Read the model definition and answer for the solid it produces. Units are mm, in the model's axes. A direction names the side the tool comes from. Coordinates: 2 decimals unless noted, no trailing zeros. Loops run counter-clockwise (first coordinate to the right, second up) from the corner with the lowest first, then second, coordinate; pieces in that order, holes last. Notation, with made-up numbers: (55, 74.25) -> (99, 74.25) arc R21 ccw to (99, 105.25) -> close; hole circle Ø4 at (2, 87). An arc over 180 degrees is marked (long way). Answer as a JSON object with one key per item and string values. Group by question number.
1) Section D-D, the plane x = 0 is taken. Give the vertices of the cut face in (y, z) (3 decimals).
2) Section C-C, the plane x = 30 is taken. Give the vertices of the cut face in (y, z).
3) Consider probe 1 along X at (y, z) = (27, 2.5); probe 2 along X at (y, z) = (0.5, 4); probe 3 along Y at (x, z) = (33.5, 5.25). Determine where each line is inside the solid, lowest interval first. Write a range as [from, to].
4) Which of the six approach directions +Z, -Z, +X, -X, +Y, -Y give full straight-line access (tool end or side, diameter ignored) to faces 4 (the face through (-3, -43, 0)), 5 (the face through (34.29, 39, 3)), 6 (the face through (-31, -38.1, 3)), 7 (the face through (31.75, 39, 3)), 8 (the face through (33, 43, 3.94))?
5) Section B-B, the plane z = 2 is taken. Count the separate pieces of the cut face and the enclosed holes in it, plus the area to 3 significant figures.
6) Determine the mould class of faces 1 (the face through (31, -38.1, 3)), 2 (the face through (38.1, -41, 3)), 3 (the face through (-1, -44.45, 3)) for opening direction Y: released by +Y, released by -Y, zero draft, split by the parting line, or undercut.
7) Flat-ended cylindrical pins translate along their axes: P1, Ø2, axis at y = -7.5, z = 2, coming from the +X side; P2, Ø3, axis at y = 45, z = 2.5, coming from the +X side; P3, Ø2, axis at y = 4, z = 4, coming from the -X side; P4, Ø1, axis at x = -2, z = 4.5, coming from the +Y side. Find the tip coordinate at first contact, or state that the pin passes through.
from build123d import *

# Parameters (mm, degrees)
SKETCH1_R            = 41.275
BOSS_EXTRUDE1_DEPTH  = 6.35
FILLET1_R            = 1.27
SKETCH2_W            = 63.5
SKETCH2_H            = 38.1
CUT_EXTRUDE1_DEPTH   = 6.35
SKETCH3_W            = 6.35
SKETCH3_H            = 25.4
BOSS_EXTRUDE2_DEPTH  = 2.54
FILLET2_R            = 1.27
FILLET2_OF_MIRROR1_R = 1.27
SKETCH6_R            = 2.54
CUT_EXTRUDE2_DEPTH   = 93.605338907


with BuildPart() as part:
    # Sketch1 → Boss-Extrude1 (new body)
    with BuildSketch(Plane.XY):
        with BuildLine():
            Line((-18.208562718, -38.1), (-38.1, -38.1))
            Line((-38.1, -38.1), (-38.1, -44.45))
            Line((-38.1, -44.45), (38.1, -44.45))
            Line((38.1, -44.45), (38.1, -38.1))
            Line((38.1, -38.1), (18.208562718, -38.1))
            ThreePointArc((18.208562718, -38.1), (0, 42.2275), (-18.208562718, -38.1))
        make_face()
        Circle(SKETCH1_R, mode=Mode.SUBTRACT)
    extrude(amount=BOSS_EXTRUDE1_DEPTH)

    # Fillet1
    fillet1_edges = [part.edges().sort_by_distance(p)[0] for p in [
        (-18.208562718, -38.1, 3.175),
        (18.208562718, -38.1, 3.175),
    ]]
    fillet(fillet1_edges, radius=FILLET1_R)

    # Sketch2 → Cut-Extrude1 (cut)
    with BuildSketch(Plane.XY.offset(6.35)):
        with Locations((0, 42.2275)):
            Rectangle(SKETCH2_W, SKETCH2_H)
    cut_extrude1 = extrude(amount=-CUT_EXTRUDE1_DEPTH, mode=Mode.SUBTRACT)

    # Sketch3 → Boss-Extrude2 (add)
    with BuildSketch(Plane(origin=(-31.75, 0, 0), x_dir=(0, 0, -1), z_dir=(1, 0, 0))):
        with Locations((-3.175, 39.073530765)):
            Rectangle(SKETCH3_W, SKETCH3_H)
    boss_extrude2 = extrude(amount=-BOSS_EXTRUDE2_DEPTH)

    # Fillet2
    # the kernel refuses this fillet: 1.27 mm, written as the material it adds along each edge
    with BuildSketch(Plane(origin=(-32.978760305, 26.373530765, 6.35), x_dir=(-0.6057595790113751, -0.7956477439394658, 0), z_dir=(0, 0, -1))) as fillet2_piece_1:
        with BuildLine():
            CenterArc((2.043961499, 1.269638951), FILLET2_R, 190.266768482, 78.366985191)
            Line((0.794296006, 1.043284905), (0.769302696, 1.038757824))
            ThreePointArc((0.769302696, 1.038757824), (0.37693855, 0.537028746), (-0.020209453, 0.015386293))
            Line((-0.020209453, 0.015386293), (0.000605618, -0.025392779))
            ThreePointArc((0.000605618, -0.025392779), (1.006840294, -0.013395128), (2.01307497, -0.025392779))
            Line((2.01307497, -0.025392779), (2.013680588, 0))
        make_face()
    extrude(amount=6.35)

    # Mirror1: Cut-Extrude1, Boss-Extrude2 across plane
    add(cut_extrude1.mirror(Plane(origin=(0, 0, 0), x_dir=(0, 0, 1), z_dir=(1, 0, 0))), mode=Mode.SUBTRACT)
    add(boss_extrude2.mirror(Plane(origin=(0, 0, 0), x_dir=(0, 0, 1), z_dir=(1, 0, 0))))

    # Fillet2 of Mirror1
    # the kernel refuses this fillet: 1.27 mm, written as the material it adds along each edge
    with BuildSketch(Plane(origin=(32.978760305, 26.373530765, 6.35), x_dir=(1, 0, 0), z_dir=(0, 0, -1))) as fillet2_of_mirror1_piece_1:
        with BuildLine():
            CenterArc((2.248334624, 0.857177399), FILLET2_OF_MIRROR1_R, 144.082725892, 78.366985191)
            Line((1.219806305, 1.602180417), (1.199235739, 1.617080477))
            ThreePointArc((1.199235739, 1.617080477), (0.59924535, 0.809204435), (-0.019836848, 0.015863778))
            Line((-0.019836848, 0.015863778), (0, -0.0254))
            ThreePointArc((0, -0.0254), (0.655619848, -0.0254), (1.292497796, -0.017143548))
            Line((1.292497796, -0.017143548), (1.311239695, 0))
        make_face()
    extrude(amount=6.35)

    # Sketch6 → Cut-Extrude2 (cut, through all)
    with BuildSketch(Plane.ZY.offset(34.29)):
        with Locations(Location((3.175, 45.423530765, 0), (0, 0, 270))):
            Circle(SKETCH6_R)
    extrude(amount=-CUT_EXTRUDE2_DEPTH, mode=Mode.SUBTRACT)


solid = part.part
Determined:
{
 "1": {"outline": "(-44.45, 0) -> (-41.275, 0) -> (-41.275, 6.35) -> (-44.45, 6.35) -> close"},
 "2": {"outline": "(-44.45, 0) -> (-38.1, 0) -> (-38.1, 6.35) -> (-44.45, 6.35) -> close; (-29.72, 0) -> (-28.35, 0) -> (-28.35, 6.35) -> (-29.72, 6.35) -> close"},
 "3": {"probe 1": "[-34.29, -31.75], [31.75, 34.29]", "probe 2": "[-42.22, -41.27], [41.27, 42.22]", "probe 3": "[-44.45, -38.1], [-25.71, -24.11], [24.11, 43.96], [46.89, 51.77]"},
 "4": {"face 4": "-Z, +X, -X, +Y, -Y", "face 5": "+Z, -Z, +X, +Y", "face 6": "+Z, -Z, -X", "face 7": "+Z, -Z, +Y", "face 8": "+X, -X"},
 "5": {"separate pieces": "3", "enclosed holes": "0", "area": "677 mm²"},
 "6": {"face 1": "undercut", "face 2": "zero draft", "face 3": "released by -Y"},
 "7": {"P1": "x = 41.72", "P2": "through", "P3": "x = -42.12", "P4": "y = -41.2"}
}
